```python
from build123d import *

# Parameters (mm, degrees)
BOSS_EXTRUDE1_DEPTH       = 14
CUT_EXTRUDE1_DEPTH        = 12
SKETCH3_W                 = 1.75
SKETCH3_H                 = 2.2
CUT_EXTRUDE2_DEPTH        = 2.25
SKETCH5_W                 = 2.2
SKETCH5_H                 = 1.25
CUT_EXTRUDE3_DEPTH        = 0.8
CHAMFER1_SIZE             = 0.3
CHAMFER1_SIZE2            = 0.173205081
CHAMFER1_OF_MIRROR1_SIZE2 = 0.3
CHAMFER1_OF_MIRROR1_SIZE  = 0.173205081
LPATTERN1_START           = -36.6
LPATTERN1_DEPTH           = 2.2
LPATTERN1_START_2         = -8.1
LPATTERN1_2_DEPTH         = 2.2
SKETCH7_W                 = 3
SKETCH7_H                 = 1.75
CUT_EXTRUDE4_DEPTH        = 2.25
CHAMFER2_SIZE             = 0.3
CHAMFER2_SIZE2            = 0.519615242
SKETCH8_W                 = 3
SKETCH8_H                 = 1.25
CUT_EXTRUDE5_DEPTH        = 0.85
CHAMFER2_OF_MIRROR2_SIZE2 = 0.519615242
CHAMFER2_OF_MIRROR2_SIZE  = 0.3
SKETCH9_W                 = 13
SKETCH9_H                 = 2
BOSS_EXTRUDE2_DEPTH       = 6
CUT_EXTRUDE9_REACH        = 54.413
SKETCH10_R                = 5.25
SKETCH11_R                = 1.5
BOSS_EXTRUDE3_DEPTH       = 14
CUT_EXTRUDE10_DEPTH       = 10
FILLET1_R                 = 2
FILLET2_R                 = 1
FILLET3_R                 = 2


# Read off the part's stored shape, not the designer's step: LPattern1
with BuildPart() as part:
    # Sketch1 → Boss-Extrude1 (new body)
    with BuildSketch(Plane(origin=(0, 3.6, 0), x_dir=(1, 0, 0), z_dir=(0, 1, 0))):
        Polygon((-13.1, -2), (-13.1, 68.428427125), (-4.928427125, 76.6), (4.928427125, 76.6), (13.1, 68.428427125), (13.1, -2), align=None)
    extrude(amount=BOSS_EXTRUDE1_DEPTH)

    # Sketch2 → Cut-Extrude1 (cut)
    with BuildSketch(Plane.XZ.offset(-3.6)):
        Polygon((11.1, -67.6), (4.1, -74.6), (-4.1, -74.6), (-11.1, -67.6), (-11.1, 0), (11.1, 0), align=None)
    extrude(amount=-CUT_EXTRUDE1_DEPTH, mode=Mode.SUBTRACT)

    # Sketch3 → Cut-Extrude2 (cut)
    with BuildSketch(Plane.XZ.offset(-3.6)):
        with Locations((10.975, -64)):
            Rectangle(SKETCH3_W, SKETCH3_H)
    cut_extrude2 = extrude(amount=-CUT_EXTRUDE2_DEPTH, mode=Mode.SUBTRACT)

    # Sketch5 → Cut-Extrude3 (cut)
    with BuildSketch(Plane.ZY.offset(-11.85)):
        with Locations((-64, 5.225)):
            Rectangle(SKETCH5_W, SKETCH5_H)
    cut_extrude3 = extrude(amount=-CUT_EXTRUDE3_DEPTH, mode=Mode.SUBTRACT)

    # Chamfer1
    chamfer1_edges = [part.edges().sort_by_distance(p)[0] for p in [
        (11.85, 3.6, -64),
    ]]
    chamfer1_side = [part.faces().sort_by_distance(p)[0] for p in [
        (11.85, 4.1, -64),
    ]]
    chamfer(chamfer1_edges, length=CHAMFER1_SIZE, length2=CHAMFER1_SIZE2, reference=chamfer1_side[0])

    # Mirror1: Cut-Extrude2, Cut-Extrude3 across plane
    add(cut_extrude2.mirror(Plane(origin=(0, 0, 0), x_dir=(0, 0, 1), z_dir=(1, 0, 0))), mode=Mode.SUBTRACT)
    add(cut_extrude3.mirror(Plane(origin=(0, 0, 0), x_dir=(0, 0, 1), z_dir=(1, 0, 0))), mode=Mode.SUBTRACT)

    # Chamfer1 of Mirror1
    chamfer1_of_mirror1_edges = [part.edges().sort_by_distance(p)[0] for p in [
        (-11.85, 3.6, -64),
    ]]
    chamfer(chamfer1_of_mirror1_edges, length=CHAMFER1_OF_MIRROR1_SIZE, length2=CHAMFER1_OF_MIRROR1_SIZE2)

    # LPattern1 outline → LPattern1 (cut)
    with BuildSketch(Plane.XY.offset(LPATTERN1_START)):
        Polygon((-12.023205081, 3.6), (-11.1, 3.6), (-11.1, 5.85), (-12.65, 5.85), (-12.65, 4.6), (-11.85, 4.6), (-11.85, 3.9), align=None)
        Polygon((11.85, 3.9), (11.85, 4.6), (12.65, 4.6), (12.65, 5.85), (11.1, 5.85), (11.1, 3.6), (12.023205081, 3.6), align=None)
    extrude(amount=LPATTERN1_DEPTH, mode=Mode.SUBTRACT)

    # LPattern1 2 outline → LPattern1 2 (cut)
    with BuildSketch(Plane.XY.offset(LPATTERN1_START_2)):
        Polygon((-12.023205081, 3.6), (-11.1, 3.6), (-11.1, 5.85), (-12.65, 5.85), (-12.65, 4.6), (-11.85, 4.6), (-11.85, 3.9), align=None)
        Polygon((11.85, 3.9), (11.85, 4.6), (12.65, 4.6), (12.65, 5.85), (11.1, 5.85), (11.1, 3.6), (12.023205081, 3.6), align=None)
    extrude(amount=LPATTERN1_2_DEPTH, mode=Mode.SUBTRACT)

    # Sketch7 → Cut-Extrude4 (cut)
    with BuildSketch(Plane.XZ.offset(-3.6)):
        with Locations((0, -74.475)):
            Rectangle(SKETCH7_W, SKETCH7_H)
    cut_extrude4 = extrude(amount=-CUT_EXTRUDE4_DEPTH, mode=Mode.SUBTRACT)

    # Chamfer2
    chamfer2_edges = [part.edges().sort_by_distance(p)[0] for p in [
        (0, 3.6, -75.35),
    ]]
    chamfer2_side = [part.faces().sort_by_distance(p)[0] for p in [
        (-12.271483253, 3.6, -33.214213562),
    ]]
    chamfer(chamfer2_edges, length=CHAMFER2_SIZE, length2=CHAMFER2_SIZE2, reference=chamfer2_side[0])

    # Sketch8 → Cut-Extrude5 (cut)
    with BuildSketch(Plane.XY.offset(-75.35)):
        with Locations((0, 5.225)):
            Rectangle(SKETCH8_W, SKETCH8_H)
    cut_extrude5 = extrude(amount=-CUT_EXTRUDE5_DEPTH, mode=Mode.SUBTRACT)

    # Mirror2: Cut-Extrude4, Cut-Extrude5 across plane
    add(cut_extrude4.mirror(Plane.XY.offset(-37.3)), mode=Mode.SUBTRACT)
    add(cut_extrude5.mirror(Plane.XY.offset(-37.3)), mode=Mode.SUBTRACT)

    # Chamfer2 of Mirror2
    chamfer2_of_mirror2_edges = [part.edges().sort_by_distance(p)[0] for p in [
        (0, 3.6, 0.75),
    ]]
    chamfer(chamfer2_of_mirror2_edges, length=CHAMFER2_OF_MIRROR2_SIZE, length2=CHAMFER2_OF_MIRROR2_SIZE2)

    # Sketch9 → Boss-Extrude2 (add)
    with BuildSketch(Plane.XZ.offset(-15.6)):
        with Locations((4.6, -50)):
            Rectangle(SKETCH9_W, SKETCH9_H)
        with Locations((4.6, -30)):
            Rectangle(SKETCH9_W, SKETCH9_H)
    extrude(amount=BOSS_EXTRUDE2_DEPTH)

    # Cut-Extrude9: up to this face of the body (flat: up to its plane)
    cut_extrude9_end = Plane(part.part.faces().sort_by_distance((4.6, 12.6, -51))[0])
    # Sketch10 → Cut-Extrude9 (cut, up to the picked face)
    with BuildSketch(Plane.XY.offset(-29), mode=Mode.PRIVATE) as cut_extrude9_sk1:
        with Locations((4.5, 9.6)):
            Circle(SKETCH10_R)
    cut_extrude9_tool1 = split(extrude(cut_extrude9_sk1.sketch, amount=-CUT_EXTRUDE9_REACH, mode=Mode.PRIVATE), bisect_by=cut_extrude9_end, keep=Keep.BOTH, mode=Mode.PRIVATE)
    add(cut_extrude9_tool1.solids().sort_by(Axis((4.5, 9.6, -29), (0, 0, -1)))[0], mode=Mode.SUBTRACT)

    # Sketch11 → Boss-Extrude3 (add)
    with BuildSketch(Plane(origin=(0, 17.6, 0), x_dir=(1, 0, 0), z_dir=(0, 1, 0))):
        with Locations(Location((-6, 20, 0), (0, 0, 270))):
            Circle(SKETCH11_R)
        with Locations(Location((-5, 58, 0), (0, 0, 270))):
            Circle(SKETCH11_R)
    extrude(amount=-BOSS_EXTRUDE3_DEPTH)

    # Sketch12 → Cut-Extrude10 (cut)
    with BuildSketch(Plane(origin=(0, 17.6, 0), x_dir=(1, 0, 0), z_dir=(0, 1, 0))):
        Polygon((-10.15, 1.25), (-10.15, -2), (10.15, -2), (10.15, 1.25), (10.15, 10.25), (-10.15, 10.25), align=None)
    extrude(amount=-CUT_EXTRUDE10_DEPTH, mode=Mode.SUBTRACT)

    # Fillet1
    fillet1_edges = [part.edges().sort_by_distance(p)[0] for p in [
        (9.014213562, 17.6, -72.514213562),
        (0, 17.6, -76.6),
        (-9.014213562, 17.6, -72.514213562),
        (-13.1, 17.6, -33.214213562),
        (-11.625, 17.6, 2),
        (11.625, 17.6, 2),
        (13.1, 17.6, -33.214213562),
    ]]
    fillet(fillet1_edges, radius=FILLET1_R)

    # Fillet2
    fillet2_edges = [part.edges().sort_by_distance(p)[0] for p in [
        (11.1, 15.6, -59.3),
        (11.1, 15.6, -14.5),
        (7.6, 15.6, -71.1),
        (11.1, 15.6, -40),
        (-7.6, 15.6, -71.1),
        (-11.1, 15.6, -33.8),
        (0, 15.6, -74.6),
    ]]
    fillet(fillet2_edges, radius=FILLET2_R)

    # Fillet3
    fillet3_edges = [part.edges().sort_by_distance(p)[0] for p in [
        (-6, 15.6, -21.5),
        (-5, 15.6, -59.5),
    ]]
    fillet(fillet3_edges, radius=FILLET3_R)


solid = part.part
```
Design review of the part built by this model. Coordinates are the model's own, in mm. A direction names the side the tool comes from. Round coordinates to 2 decimals unless told otherwise and drop trailing zeros. Order: outer loops, then holes, each group sorted by start corner. A loop starts at its lowest first (then second) coordinate and runs counter-clockwise, first axis right, second up. Notation, with made-up numbers: (6.25, 62) - (65.25, 62) arc R24 cw to (65.25, 79) - close; hole circle Ø6 at (-9.75, -26). An arc over 180 degrees is marked (long way). One line per question, with ' | ' between items.
Item 1: Draft analysis for pull direction Y (two halves, no side actions). For faces 1 (the face through (8.65, 17.03, -72.03)), 2 (the face through (0, 9, -74.6)), 3 (the face through (-1.5, 5, -75)), state which applies: +Y half, -Y half, draft (parallel to the pull), parting line (faces both ways), or undercut.
Checks:
face 1: +Y half | face 2: draft | face 3: undercut
Item 2: Take a section at B-B, the plane z = -37.5. Write out the cut boundary in (x, y), then the cut area to 3 significant figures.
Checks:
outline: (-13.1, 3.6) - (-11.1, 3.6) - (-11.1, 14.6) arc R1 cw to (-10.1, 15.6) - (10.1, 15.6) arc R1 cw to (11.1, 14.6) - (11.1, 3.6) - (13.1, 3.6) - (13.1, 15.6) arc R2 ccw to (11.1, 17.6) - (-11.1, 17.6) arc R2 ccw to (-13.1, 15.6) - close | area: 99.1 mm²
Item 3: Machinability: for faces 4 (the face through (-13.1, 10, -33)), 5 (the face through (-9.07, 9.52, -72.46)), 6 (the face through (12, 5, -8.1)), 7 (the face through (10.15, 16, -3)), 8 (the face through (7.6, 9, -71.1)), which of the approach directions +Z, -Z, +X, -X, +Y, -Y give a long, thin tool a straight path to every point of the face, cutting with its end or side? Answer none if there is none.
Checks:
face 4: +Z, -Z, -X, +Y, -Y | face 5: -Z, -X, +Y, -Y | face 6: none | face 7: +Z, +Y | face 8: -Y
Item 4: Take a section at A-A, the plane z = -20. Write out the cut boundary in (x, y).
Checks:
outline: (-13.1, 3.6) - (-11.1, 3.6) - (-11.1, 14.6) arc R1 cw to (-10.1, 15.6) - (-9.5, 15.6) arc R2 cw to (-7.5, 13.6) - (-7.5, 3.6) - (-4.5, 3.6) - (-4.5, 13.6) arc R2 cw to (-2.5, 15.6) - (10.1, 15.6) arc R1 cw to (11.1, 14.6) - (11.1, 3.6) - (13.1, 3.6) - (13.1, 15.6) arc R2 ccw to (11.1, 17.6) - (-11.1, 17.6) arc R2 ccw to (-13.1, 15.6) - close
Item 5: For P1, Ø0.5, axis at x = -11.5, z = -35.5, coming from the -Y side; P2, Ø10, axis at x = 1.5, z = -49.5, coming from the -Y side; P3, Ø10, axis at x = -3, z = -43.5, coming from the -Y side, all flat-tipped, find the tip position at first contact; note any pin that passes through.
Checks:
P1: y = 5.85 | P2: y = 9.6 | P3: y = 15.6
Item 6: Wall thickness on line 1 (Z direction, x = -2, y = 6.5); line 2 (X direction, y = 14.75, z = -1.5); line 3 (Z direction, x = -5, y = 14): over which ranges is each line inside the solid? List them lowest first. Write a range as [from, to].
Checks:
line 1: [-76.6, -74.6], [0, 2] | line 2: [-13.1, -11.09], [11.09, 13.1] | line 3: [-76.53, -73.7], [-59.54, -56.46], [-21.17, -18.83]
